Design review of the part built by this model. Coordinates are the model's own, in mm. Face numbers are marked on the shaded views. Coordinates: 2 decimals unless noted, no trailing zeros. Loops run counter-clockwise (first coordinate to the right, second up) from the corner with the lowest first, then second, coordinate; pieces in that order, holes last. Notation, with made-up numbers: M -38.5,23 L 4.5,23 A10 ccw 4.5,30 Z; hole C 25.5,-33 d1. An arc over 180 degrees is marked long. One line per item, written item: value.
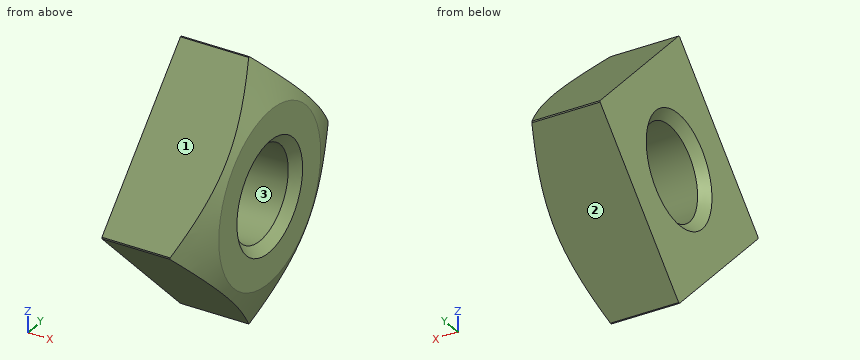
Autodesk Inventor part; units mm, degrees
ref_plane "IP1_XY" through (0, 0, 0) normal (1, 0, 0) x (0, 0, -1)
ref_plane "IP1_YZ" through (0, 0, 0) normal (0, 0, -1) x (0, 1, 0)
ref_plane "IP1_ZX" through (0, 0, 0) normal (0, 1, 0) x (1, 0, 0)
sketch "Sketch_2" plane through (0, 0, 0) normal (0, 0, 1) x (1, 0, 0)
  line L0 (8, 0) -> (0, 0)
  line L1 (0, 0) -> (0, 12.0208)
  line L2 (0, 12.0208) -> (6.143, 12.0208)
  line L3 (6.143, 12.0208) -> (8, 7.75)
  line L4 (8, 7.75) -> (8, 0)
  line L5 (8, 0) -> (0, 0)
revolve "Revolution1" add sketch "Sketch_2" angle 360 about axis through (8, 0, 0) along (1, 0, 0)
sketch "Skizze_2" plane through (0, 0, 0) normal (1, 0, 0) x (0, 1, 0)
  line L0 (34, 34) -> (-34, 34)
  line L1 (-34, 34) -> (-34, -34)
  line L2 (-34, -34) -> (34, -34)
  line L3 (34, -34) -> (34, 34)
  line L4 (0, 12.0915) -> (-12.0915, 0)
  line L5 (-12.0915, 0) -> (0, -12.0915)
  line L6 (0, -12.0915) -> (12.0915, 0)
  line L7 (12.0915, 0) -> (0, 12.0915)
extrude "Extrusion1" cut sketch "Skizze_2" along normal blind 8
sketch "Sketch_1" plane through (0, 0, 0) normal (0, 0, 1) x (1, 0, 0)
  line L0 (8, 0) -> (0, 0)
  line L1 (0, 0) -> (0, 5)
  line L2 (0, 5) -> (0.812, 4.188)
  line L3 (0.812, 4.188) -> (7.188, 4.188)
  line L4 (7.188, 4.188) -> (8, 5)
  line L5 (8, 5) -> (8, 0)
  line L6 (8, 0) -> (0, 0)
revolve "Revolution2" cut sketch "Sketch_1" angle 360 about axis through (8, 0, 0) along (1, 0, 0)
thread "Thread1"
ref_plane "IP1_XY" through (0, 0, 0) normal (1, 0, 0) x (0, 0, -1)
ref_plane "IP1_YZ" through (0, 0, 0) normal (0, 0, -1) x (0, 1, 0)
ref_plane "IP1_ZX" through (0, 0, 0) normal (0, 1, 0) x (1, 0, 0)
ref_plane "IP2_XY" through (8, 0, 0) normal (1, 0, 0) x (0, 0, -1)
ref_plane "IP2_YZ" through (8, 0, 0) normal (0, 0, -1) x (0, 1, 0)
ref_plane "IP2_ZX" through (8, 0, 0) normal (0, 1, 0) x (1, 0, 0)
properties part number "DIN 557 - M10"
(1) To check wall thickness, follow line 1 along Z through (x, y) = (5.25, 0); line 2 along Y through (x, z) = (0.75, 2); line 3 along Z through (x, y) = (2, 2.25). State the ranges of each line that lie inside material, in increasing order. Write a range as [from, to].
Reply:
line 1: z = [-12.02, -4.19], [4.19, 12.02]
line 2: y = [-10.09, -3.75], [3.75, 10.09]
line 3: z = [-9.84, -3.53], [3.53, 9.84]
(2) Insertion check: pin 1 (4 mm diameter, centred on x = 6.5, y = -4, fed in from -Z); pin 2 (1 mm diameter, centred on x = 3.5, z = 8.5, fed in from -Y); pin 3 (4 mm diameter, centred on x = 2, z = 5.5, fed in from -Y); pin 4 (4 mm diameter, centred on y = 9, z = -2.5, fed in from +X). Each pin has a flat end and moves straight along its axis. Give the tip position at first contact, or say it passes through.
Reply:
pin 1: stops at z = -10.09
pin 2: stops at y = -4.09
pin 3: stops at y = -8.59
pin 4: stops at x = 8
(3) Mouldability with a two-part tool opening along Y and no side actions: class the marked faces 1, 2 and 3 as released by +Y, released by -Y, zero draft, split by the parting line, or undercut.
Reply:
face 1: released by -Y
face 2: released by +Y
face 3: undercut
(4) We need section A-A on x = 5.5. State the section outline as (y, z) points, then the cut area to 3 significant figures.
Reply:
outline: M -12.02,-0.07 L -0.07,-12.02 A12.02 ccw 0.07,-12.02 L 12.02,-0.07 A12.02 ccw 12.02,0.07 L 0.07,12.02 A12.02 ccw -0.07,12.02 L -12.02,0.07 A12.02 ccw Z; hole C 0,0 d8.38
area: 237 mm2
